Input: part model. Units: mm. Frame: model coordinates. A direction names the side the tool comes from. Coordinates: 2 decimals unless noted, no trailing zeros. Loops run counter-clockwise (first coordinate to the right, second up) from the corner with the lowest first, then second, coordinate; pieces in that order, holes last. Notation, with made-up numbers: (67, -37) -> (72, -37) arc R27 ccw to (72, -3) -> close; hole circle Ø7 at (22, 39.5). An arc over 180 degrees is marked (long way). Answer as a JSON object with one key per item and string values.
Autodesk Inventor part; units mm, degrees
ref_plane "YZ Plane" through (0, 0, 0) normal (1, 0, 0) x (0, 1, 0)
ref_plane "XZ Plane" through (0, 0, 0) normal (0, 1, 0) x (-1, 0, 0)
ref_plane "XY Plane" through (0, 0, 0) normal (0, 0, 1) x (1, 0, 0)
sketch "Sketch1" plane through (0, 0, 0) normal (0, 1, 0) x (-1, 0, 0)
  line L0 (0, 0) -> (-12, 0)
  line L1 (-12, 0) -> (-12, -40)
  line L2 (-12, -40) -> (0, -40)
  line L3 (0, -40) -> (0, 0)
  point P0 (-6, 0)
  dimension "d0" = 40
  dimension "d1" = 12
extrude "Extrusion1" add sketch "Sketch1" along normal blind 40
sketch "Sketch2" plane through (12, 0, -40) normal (0, 0, -1) x (-1, 0, 0)
  line L0 (0, 40) -> (12, 40)
  line L1 (8, 40) -> (8, 4)
  line L2 (8, 4) -> (4, 4)
  line L3 (4, 4) -> (7.129, 36.8805)
  line L4 (7.129, 36.8805) -> (4, 40)
  line L5 (4, 40) -> (8, 40)
  line L6 (12, 0) -> (12, 40)
  line L7 (0, 0) -> (0, 40)
  line L8 (0, 0) -> (12, 0)
  line L9 (0, 4) -> (3.129, 36.8805)
  line L10 (3.129, 36.8805) -> (0, 40)
  point P0 (6, 0)
  point P1 (6, 4)
  dimension "d4" = 4
  dimension "d5" = 4
  dimension "d6" = 4
  dimension "d7" = 4
  dimension "d8" = 4
  dimension "d9" = 4
  dimension "d10" = 3.982
  dimension "d11" = 2.8241
extrude "Extrusion2" cut sketch "Sketch2" against normal blind 40 contours L10 L9 L7 | L0 L1 L2 L3 L4
fillet "Fillet1" radius 2 6 edges at (12, 0, -20) (0, 0, -20) (0, 40, -20) (4, 40, -20) (8, 40, -20) (4.871, 36.8805, -20)
sketch "Sketch3" plane through (0, 2, -40) normal (-1, 0, 0) x (0, 0, 1)
  line L0 (40, 0) -> (0, 0)
  line L1 (39, 0) -> (1, 0)
  line L2 (1, 0) -> (1, 10)
  line L3 (1, 10) -> (39, 10)
  line L4 (39, 10) -> (39, 0)
  line L5 (0, 0) -> (0, 36)
  point P0 (40, -2)
  point P1 (1, 0)
  dimension "d15" = 38
  dimension "d16" = 1
  dimension "d17" = 10
extrude "Extrusion3" add sketch "Sketch3" along normal blind 14
sketch "Sketch4" plane through (-14, 2, -1) normal (0, -1, 0) x (1, 0, 0)
  circle A0 centre (7, -7) radius 5
  circle A1 centre (7, -31) radius 5
  circle A2 centre (7, -19) radius 5
  line L0 (14, -38) -> (0, -38)
  line L1 (0, -38) -> (0, 0)
  point P0 (14, 1)
  point P1 (0, -19)
  dimension "d20" = 10
  dimension "d21" = 10
  dimension "d22" = 10
  dimension "d23" = 2
  dimension "d24" = 2
  dimension "d25" = 2
  dimension "d26" = 7
  dimension "d27" = 7
  dimension "d28" = 7
extrude "Extrusion4" cut sketch "Sketch4" against normal blind 14
fillet "Fillet2" radius 7 1 edges at (-14, 7, -39)
fillet "Fillet3" radius 7 1 edges at (-14, 7, -1)
sketch "Sketch5" plane through (0, 2, -39) normal (0, -1, 0) x (1, 0, 0)
  circle A0 centre (-7, 19) radius 5
  arc A1 (-14, 7) -> (-7, 0) centre (-7, 7) ccw
  arc A2 (-10.6056, 13) -> (-14, 7) centre (-7, 7) ccw
  line L0 (-14, 7) -> (-14, 31)
  circle A3 centre (-7, 7) radius 5
  arc A4 (-14, 19) -> (-10.6056, 13) centre (-7, 19) ccw
  circle A5 centre (-7, 31) radius 5
  arc A6 (-10.6056, 25) -> (-14, 19) centre (-7, 19) ccw
  arc A7 (-7, 38) -> (-14, 31) centre (-7, 31) ccw
  arc A8 (-14, 31) -> (-10.6056, 25) centre (-7, 31) ccw
  line L1 (-14, 31) -> (-14, 7)
  point P0 (0, 39)
  dimension "d33" = 7
  dimension "d34" = 7
extrude "Extrusion5" cut sketch "Sketch5" against normal blind 14 contours L0 A8 A6 | A2 L0 A4
properties part number "theWritersHolster"
1. Access query for faces 4 (the face through (0.57, 0.6, -19.72)), 5 (the face through (-3, 7, -39)), 6 (the face through (3.43, 39.4, -19.72)), 7 (the face through (0.6, 39.43, -19.72)), 8 (the face through (10.414, 38.418, -20.28)). Directions: +Z, -Z, +X, -X, +Y, -Y. A direction counts if a zero-diameter tool reaches every point of the face in a straight line with its end or side. Return the directions, or none.
Reply:
{"face 4": "+Z, -Z, -X, -Y", "face 5": "-Z, -X, +Y, -Y", "face 6": "+Z, -Z, +Y", "face 7": "+Z, -Z, -X, +Y", "face 8": "+Z, -Z, +X"}
2. Section query A-A (x = -2.75). Return loops of the section in (y, z).
Reply:
{"outline": "(2, -39) -> (12, -39) -> (12, -34.63) -> (2, -34.63) -> close; (2, -29.37) -> (12, -29.37) -> (12, -22.63) -> (2, -22.63) -> close; (2, -17.37) -> (12, -17.37) -> (12, -10.63) -> (2, -10.63) -> close; (2, -5.37) -> (12, -5.37) -> (12, -1) -> (2, -1) -> close"}
3. Section query C-C (y = 19). Return loops of the section in (x, z), plus the area to 3 significant figures.
Reply:
{"outline": "(0, -40) -> (4, -40) -> (4, 0) -> (0, 0) -> close; (6.57, -40) -> (10.57, -40) -> (10.57, 0) -> (6.57, 0) -> close", "area": "320 mm2"}
4. Pin query (flat end, axial travel): P1, Ø2, axis at x = -4.5, y = 5, coming from the -Z side; P2, Ø11.5, axis at x = -7, z = -20, coming from the -Y side; P3, Ø5, axis at x = -4, y = 31, coming from the +Z side; P4, Ø10, axis at x = -7.5, y = 4.5, coming from the +Z side. Return the tip coordinate at first contact, or that it passes through.
Reply:
{"P1": "stops at z = -39", "P2": "stops at y = 2", "P3": "passes through", "P4": "stops at z = -1"}
5. Mould query, pull axis Y, two halves, no side actions, for faces 1 (the face through (6, 4, -20)), 2 (the face through (-2.23, 6.93, -6.5)), 3 (the face through (10, 40, -20)). Classes: pulls with the +Y half, pulls with the -Y half, needs draft (parallel to the pull), parting line crosses it, or undercut.
Reply:
{"face 1": "undercut", "face 2": "needs draft", "face 3": "pulls with the +Y half"}
6. Line query: line 1 along Z through (x, y) = (-7, 4.75); line 2 along Z through (x, y) = (-3.5, 9.5); line 3 along Y through (x, z) = (-8.75, -25). Output: solid intervals per line, ascending.
Reply:
{"line 1": "z = -39 to -37, -27 to -25, -15 to -13, -3 to -1", "line 2": "z = -39 to -35.57, -28.43 to -23.57, -16.43 to -11.57, -4.43 to -1", "line 3": "y = 2 to 12"}
7. Section query B-B (y = 7). Return loops of the section in (x, z).
Reply:
{"outline": "(-14, -32) arc R7 ccw to (-7, -39) -> (0, -39) -> (0, -40) -> (4, -40) -> (4, 0) -> (0, 0) -> (0, -1) -> (-7, -1) arc R7 ccw to (-14, -8) arc R7 ccw to (-10.61, -14) arc R7 ccw to (-14, -20) arc R7 ccw to (-10.61, -26) arc R7 ccw to start; (7.71, -40) -> (11.71, -40) -> (11.71, 0) -> (7.71, 0) -> close; hole circle Ø10 at (-7, -32); hole circle Ø10 at (-7, -20); hole circle Ø10 at (-7, -8)"}
